Part model, mm, in its own coordinate system. A direction names the side the tool comes from. Round coordinates to 2 decimals unless told otherwise and drop trailing zeros. Loops run counter-clockwise (first coordinate to the right, second up) from the corner with the lowest first, then second, coordinate; pieces in that order, holes last. Notation, with made-up numbers: M 36.5,-4 L 81.5,-4 A20 cw 81.5,35 Z; hole C 84,77.25 d5. An arc over 180 degrees is marked long. Answer as CSV lines item,"result". Start each with the question number.
Item 1: Which spindle directions (+Z, -Z, +X, -X, +Y, -Y) get a long thin tool onto all of the face, cutting with end or side? Do faces 1 (the flat face through (0, 0, -4)), 2 (the cylindrical face through (1, 0.32, 1.18)). Say none if no direction does.
Item 2: Wall check: line 1 (Y direction, x = 0, z = -3); line 2 (Z direction, x = 0.9, y = 0.2); line 3 (Y direction, x = 0.7, z = 0). Give the ranges that are in metal, low to high.
Item 3: Drop a flat-ended pin along its axis: pin 1 Ø1 at (x, y) = (1, -0.5) entering from +Z. Give the stop position or say it passes through.
Item 4: Band-saw the part on A-A (z = 5.25). Give the cut face in (x, y), and give its area (3 significant figures).
```python
from build123d import *

# Parameters (mm, degrees)
DODANIE_WYCI_GNI_CIE1_DEPTH      = 6.5
DODANIE_WYCI_GNI_CIE1_DEPTH_BACK = 4
SZKIC1_R                         = 1.05
SZKIC2_R                         = 1.55
DODANIE_WYCI_GNI_CIE2_DEPTH      = 1
ZAOKR_GLENIE1_R                  = 1.55


with BuildPart() as part:
    # Szkic1 → Dodanie-wyciągnięcie1 (new, two sides: drawn at the far end of the back side and taken through both)
    with BuildSketch(Plane.XY.offset(-DODANIE_WYCI_GNI_CIE1_DEPTH_BACK)):
        Circle(SZKIC1_R)
    extrude(amount=DODANIE_WYCI_GNI_CIE1_DEPTH + DODANIE_WYCI_GNI_CIE1_DEPTH_BACK)

    # Szkic2 → Dodanie-wyciągnięcie2 (add)
    with BuildSketch(Plane.XY.offset(6.5)):
        Circle(SZKIC2_R)
    extrude(amount=DODANIE_WYCI_GNI_CIE2_DEPTH)

    # Zaokrąglenie1
    # the kernel refuses this fillet: 1.55 mm, written as the material it takes off along each edge
    with BuildSketch(Plane(origin=(0, 0, 7.5), x_dir=(1, 0, 0), z_dir=(0, -1, 0))) as zaokr_glenie1_piece_1:
        with BuildLine():
            CenterArc((0.100862325, -1.55), ZAOKR_GLENIE1_R, 20.783559596, 69.216440404)
            Line((0.100862325, 0), (0.100862325, 0.031))
            Line((0.100862325, 0.031), (1.55, 0.031))
            Line((1.55, 0.031), (1.581, 0))
            ThreePointArc((1.581, 0), (1.581, -0.5), (1.578982753, -0.989))
            Line((1.578982753, -0.989), (1.55, -1))
        make_face()
    revolve(axis=Axis((0, 0, 7.5), (0, 0, 1)), mode=Mode.SUBTRACT)


solid = part.part
```
Answer block:
1,face 1,"-Z, +X, -X, +Y, -Y"
1,face 2,"-Z"
2,line 1,"y = -1.05 to 1.05"
2,line 2,"z = -4 to 7.26"
2,line 3,"y = -0.78 to 0.78"
3,pin 1,"stops at z = 7.41"
4,outline,"C 0,0 d2.1"
4,area,"3.46 mm^2"
